```python
from build123d import *

# Parameters (mm, degrees)
PAD_DEPTH = 5


with BuildPart() as part:
    # Sketch → Pad (new body)
    with BuildSketch(Plane.XY):
        Polygon((-2.215162, 59.759811), (-2.215162, -3.075415), (38.48941, -3.075415), (45.010048, 28.539799), (36.908657, 47.508923), (23.274607, 59.759811), align=None)
        Polygon((0, 0), (35, 0), (37, 7.2), (38.5, 14.4), (39.6, 21.6), (39.7, 28.8), (38.4, 36), (35.3, 43.2), (30.5, 50.4), (20, 57.6), (0, 57.6), align=None, mode=Mode.SUBTRACT)
    extrude(amount=PAD_DEPTH)


solid = part.part
```
Design review of the part built by this model. Coordinates are the model's own, in mm. A direction names the side the tool comes from. Give positions to 0.01 mm unless a question says otherwise; leave off trailing zeros. Loops run counter-clockwise (first coordinate to the right, second up) from the corner with the lowest first, then second, coordinate; pieces in that order, holes last. Notation, with made-up numbers: (72.5, -31.5) -> (91.5, -31.5) arc R27 ccw to (91.5, 4.5) -> close; hole circle Ø3 at (-25, 73). An arc over 180 degrees is marked (long way). Write each question's results on one line, items separated by ' | '.
Q1. Machinability: for faces 1 (the face through (11, 59.76, 2)), 2 (the face through (36.87, 39.55, 2.46)), which of the approach directions +Z, -Z, +X, -X, +Y, -Y give a long, thin tool a straight path to every point of the face, cutting with its end or side? Answer none if there is none.
Reply:
face 1: +Z, -Z, +X, -X, +Y | face 2: +Z, -Z
Q2. Take a section at D-D, the plane x = 41. Write out the cut boundary in (y, z), plus the area to 3 significant figures.
Reply:
outline: (9.1, 0) -> (37.93, 0) -> (37.93, 5) -> (9.1, 5) -> close | area: 144 mm²
Q3. Wall thickness on L1, parallel to Y at x = 17.5, z = 3.2; L2, parallel to X at y = 28.5, z = 3.25; L3, parallel to Y at x = 22, z = 1.1: over which ranges is each line inside the solid? List them lowest first.
Reply:
L1: y = -3.08 to 0, 57.6 to 59.76 | L2: x = -2.22 to 0, 39.7 to 45 | L3: y = -3.08 to 0, 56.23 to 59.76
Q4. The part is to be moulded in two halves that separate along Y. For faces 3 (the face through (17, 0, 2)), 4 (the face through (-2.215, 29, 2)), 5 (the face through (41.7, 12.5, 2.5)), say which applies: +Y half, -Y half, draft (parallel to the pull), parting line (faces both ways), or undercut.
Reply:
face 3: undercut | face 4: draft | face 5: -Y half
Q5. Take a section at A-A, the plane z = 3.55. Write out the cut boundary in (x, y), plus the area to 3 significant figures.
Reply:
outline: (-2.22, -3.08) -> (38.49, -3.08) -> (45.01, 28.54) -> (36.91, 47.51) -> (23.27, 59.76) -> (-2.22, 59.76) -> close; hole (0, 0) -> (35, 0) -> (37, 7.2) -> (38.5, 14.4) -> (39.6, 21.6) -> (39.7, 28.8) -> (38.4, 36) -> (35.3, 43.2) -> (30.5, 50.4) -> (20, 57.6) -> (0, 57.6) -> close | area: 542 mm²
Q6. Take a section at C-C, the plane x = 22. Write out the cut boundary in (y, z).
Reply:
outline: (-3.08, 0) -> (0, 0) -> (0, 5) -> (-3.08, 5) -> close; (56.23, 0) -> (59.76, 0) -> (59.76, 5) -> (56.23, 5) -> close
Q7. Take a section at B-B, the plane y = 16.5. Write out the cut boundary in (x, z).
Reply:
outline: (-2.22, 0) -> (0, 0) -> (0, 5) -> (-2.22, 5) -> close; (38.82, 0) -> (42.53, 0) -> (42.53, 5) -> (38.82, 5) -> close
Q8. For pin 1 Ø3 at (y, z) = (45, 1) entering from +X; pin 2 Ø6 at (x, y) = (34, 18) entering from -Z, all flat-tipped, find the tip position at first contact; note any pin that passes through.
Reply:
pin 1: stops at x = 38.62 | pin 2: passes through
